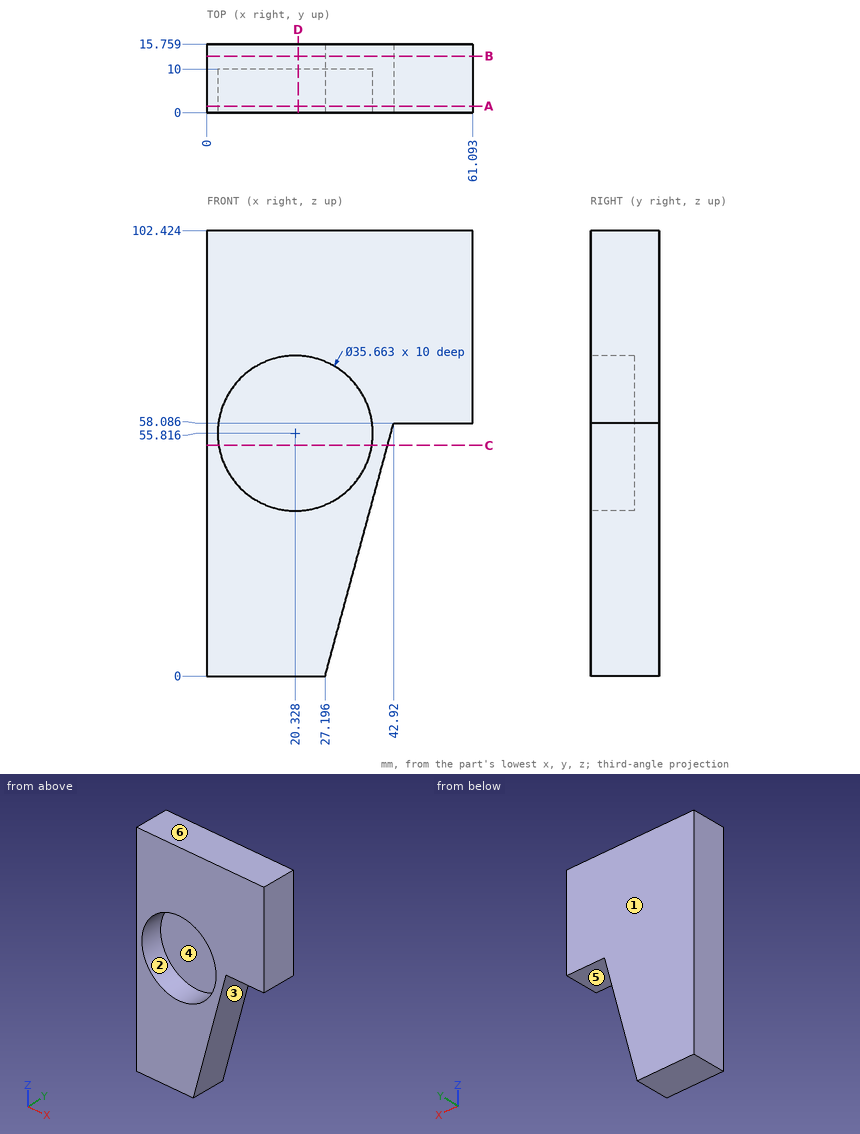
For this review, use the dimensioned drawing (mm, ordinates from the lowest corner) and the shaded views. A direction names the side the tool comes from. Give positions to 0.01 mm unless a question says otherwise; leave off trailing zeros. Write each loop counter-clockwise with the first axis right and the second up, starting at its lowest first coordinate (ties: lowest second). Pieces come first, ordered by that corner, then holes. Notation, with made-up numbers: M 15.5,-4.5 L 38.5,-4.5 A21 ccw 38.5,29.5 Z; hole C 63.25,37 d11. An arc over 180 degrees is marked long. Answer as a JSON object with one key per item and string values. Group by question number.
Item 1: Consider section C-C on z = 53. Write out the cut boundary in (x, y) (1 decimal).
Item 2: For probe 1 along Z at (x, y) = (45, 5) (1 decimal); probe 2 along Y at (x, z) = (23, 38.5); probe 3 along X at (y, z) = (7.75, 69.5) (1 decimal), list the stretches that pass through material, from the lowest coordinate up. Write a range as [from, to].
Item 3: For pin 1 Ø10.5 at (x, z) = (28.5, 56) entering from -Y; pin 2 Ø1.5 at (y, z) = (10, 47) entering from +X; pin 3 Ø5 at (x, y) = (52, 4) entering from -Z, all flat-tipped, find the tip position at first contact; note any pin that passes through.
Item 4: Tool access review of the marked faces 5 and 6: name each direction out of +Z, -Z, +X, -X, +Y, -Y from which nothing blocks a thin tool from reaching the whole face with its end or side.
Item 5: Consider section D-D on x = 21. Write out the cut boundary in (y, z) (1 decimal).
Item 6: Consider section A-A on y = 1.5. Write out the cut boundary in (x, z) (1 decimal).
Item 7: Consider section B-B on y = 13. Write out the cut boundary in (x, z) (1 decimal).
Item 8: Draft analysis for pull direction X (two halves, no side actions). For the marked faces 1, 2, 3 and 4, state which applies: +X half, -X half, draft (parallel to the pull), parting line (faces both ways), or undercut.
Check result:
{
 "1": {"outline": "M 0,0 L 2.7,0 L 2.7,10 L 37.9,10 L 37.9,0 L 41.5,0 L 41.5,15.8 L 0,15.8 Z"},
 "2": {"probe 1": "z = [58.1, 102.4]", "probe 2": "y = [10, 15.76]", "probe 3": "x = [0, 8.9], [31.8, 61.1]"},
 "3": {"pin 1": "stops at y = 10", "pin 2": "stops at x = 40.12", "pin 3": "stops at z = 58.09"},
 "4": {"face 5": "-Z, +X, +Y, -Y", "face 6": "+Z, +X, -X, +Y, -Y"},
 "5": {"outline": "M 0,0 L 15.8,0 L 15.8,102.4 L 0,102.4 L 0,73.6 L 10,73.6 L 10,38 L 0,38 Z"},
 "6": {"outline": "M 0,0 L 27.2,0 L 42.9,58.1 L 61.1,58.1 L 61.1,102.4 L 0,102.4 Z; hole C 20.3,55.8 d35.7"},
 "7": {"outline": "M 0,0 L 27.2,0 L 42.9,58.1 L 61.1,58.1 L 61.1,102.4 L 0,102.4 Z"},
 "8": {"face 1": "draft", "face 2": "undercut", "face 3": "+X half", "face 4": "undercut"}
}
